```python
from build123d import *

# Parameters (mm, degrees)
SKETCH17_R              = 35
SKETCH18_R              = 60
BOSS_EXTRUDE2_DEPTH     = 10
SKETCH19_R              = 60
BOSS_EXTRUDE3_DEPTH     = 10
CUT_EXTRUDE1_DEPTH      = 153.968934548
CUT_EXTRUDE1_DEPTH_BACK = 10
SKETCH20_R              = 4
SKETCH21_R              = 25
CUT_EXTRUDE3_DEPTH      = 153.968934548
CUT_EXTRUDE3_DEPTH_BACK = 10
SKETCH21_3_R            = 25
SKETCH22_R              = 25
CUT_EXTRUDE10_DEPTH     = 10
CUT_EXTRUDE11_START     = 10
SKETCH22_3_R            = 25
CUT_EXTRUDE11_DEPTH     = 10
SKETCH24_R              = 4
CUT_EXTRUDE18_DEPTH     = 10


with BuildPart() as part:
    # Sweep1: sweep along a path in Sketch16
    with BuildLine(Plane(origin=(0, 0, 0), x_dir=(0, 0, -1), z_dir=(1, 0, 0))) as sweep1_path:
        ThreePointArc((0, 0), (-7.612046749, 38.268343237), (-29.289321881, 70.710678119))
    # Sketch17 → Sweep1 (sweep)
    with BuildSketch(Plane(origin=(0, 0, 0), x_dir=(1, 0, 0), z_dir=(0, 1, 0))):
        with Locations((0, -29.289321881)):
            Circle(SKETCH17_R)
    sweep(path=sweep1_path.line)

    # Sketch18 → Boss-Extrude2 (add)
    with BuildSketch(Plane(origin=(0, 0, 0), x_dir=(-1, 0, 0), z_dir=(0, -1, 0))):
        with Locations(Location((0, -29.289321881, 0), (0, 0, 90))):
            Circle(SKETCH18_R)
    extrude(amount=BOSS_EXTRUDE2_DEPTH)

    # Sketch19 → Boss-Extrude3 (add)
    with BuildSketch(Plane(origin=(0, 50, 50), x_dir=(1, 0, 0), z_dir=(0, 0.7071067811865513, 0.7071067811865438))):
        with Locations(Location((0, 0, 0), (0, 0, 270))):
            Circle(SKETCH19_R)
    extrude(amount=BOSS_EXTRUDE3_DEPTH)

    # Sketch20 → Cut-Extrude1 (cut, two sides: drawn at the far end of the back side and taken through both)
    with BuildSketch(Plane(origin=(0, 0, 0), x_dir=(-1, 0, 0), z_dir=(0, -1, 0)).offset(-CUT_EXTRUDE1_DEPTH_BACK)):
        with Locations(Location((0, 20.710678119, 0), (0, 0, 90))):
            Circle(SKETCH20_R)
        with Locations(Location((25, 14.011948308, 0), (0, 0, 90))):
            Circle(SKETCH20_R)
        with Locations(Location((43.301270189, -4.289321881, 0), (0, 0, 90))):
            Circle(SKETCH20_R)
        with Locations(Location((50, -29.289321881, 0), (0, 0, 90))):
            Circle(SKETCH20_R)
        with Locations(Location((43.301270189, -54.289321881, 0), (0, 0, 90))):
            Circle(SKETCH20_R)
        with Locations(Location((25, -72.590592071, 0), (0, 0, 90))):
            Circle(SKETCH20_R)
        with Locations(Location((0, -79.289321881, 0), (0, 0, 90))):
            Circle(SKETCH20_R)
        with Locations(Location((-25, -72.590592071, 0), (0, 0, 90))):
            Circle(SKETCH20_R)
        with Locations(Location((-43.301270189, -54.289321881, 0), (0, 0, 90))):
            Circle(SKETCH20_R)
        with Locations(Location((-50, -29.289321881, 0), (0, 0, 90))):
            Circle(SKETCH20_R)
        with Locations(Location((-43.301270189, -4.289321881, 0), (0, 0, 90))):
            Circle(SKETCH20_R)
        with Locations(Location((-25, 14.011948308, 0), (0, 0, 90))):
            Circle(SKETCH20_R)
    extrude(amount=CUT_EXTRUDE1_DEPTH + CUT_EXTRUDE1_DEPTH_BACK, mode=Mode.SUBTRACT)

    # Cut-Sweep2: sweep along a path in Sketch16<3>
    with BuildLine(Plane(origin=(0, 0, 0), x_dir=(0, 0, -1), z_dir=(1, 0, 0))) as cut_sweep2_path:
        ThreePointArc((0, 0), (-7.612046749, 38.268343237), (-29.289321881, 70.710678119))
    # Sketch21 → Cut-Sweep2 (sweep, cut)
    with BuildSketch(Plane(origin=(0, 0, 0), x_dir=(-1, 0, 0), z_dir=(0, -1, 0))):
        with Locations((0, -29.289321881)):
            Circle(SKETCH21_R)
    sweep(path=cut_sweep2_path.line, mode=Mode.SUBTRACT)

    # Sketch21<3> → Cut-Extrude3 (cut, two sides: drawn at the far end of the back side and taken through both)
    with BuildSketch(Plane(origin=(0, 0, 0), x_dir=(-1, 0, 0), z_dir=(0, -1, 0)).offset(-CUT_EXTRUDE3_DEPTH_BACK)):
        with Locations(Location((0, -29.289321881, 0), (0, 0, 180.810311696))):
            Circle(SKETCH21_3_R)
    extrude(amount=CUT_EXTRUDE3_DEPTH + CUT_EXTRUDE3_DEPTH_BACK, mode=Mode.SUBTRACT)

    # Sketch22 → Cut-Extrude10 (cut)
    with BuildSketch(Plane(origin=(0, 50, 50), x_dir=(1, 0, 0), z_dir=(0, 0.7071067811865513, 0.7071067811865438))):
        Circle(SKETCH22_R)
    extrude(amount=-CUT_EXTRUDE10_DEPTH, mode=Mode.SUBTRACT)

    # Sketch22<3> → Cut-Extrude11 (cut)
    with BuildSketch(Plane(origin=(0, 50, 50), x_dir=(1, 0, 0), z_dir=(0, 0.7071067811865513, 0.7071067811865438)).offset(CUT_EXTRUDE11_START)):
        with Locations(Location((0, 0, 0), (0, 0, 270))):
            Circle(SKETCH22_3_R)
    extrude(amount=-CUT_EXTRUDE11_DEPTH, mode=Mode.SUBTRACT)

    # Sketch24 → Cut-Extrude18 (cut)
    with BuildSketch(Plane(origin=(0, 50, 50), x_dir=(1, 0, 0), z_dir=(0, 0.7071067811865513, 0.7071067811865438))):
        with Locations(Location((0, 50, 0), (0, 0, 270))):
            Circle(SKETCH24_R)
        with Locations(Location((25, 43.301270189, 0), (0, 0, 270))):
            Circle(SKETCH24_R)
        with Locations(Location((43.301270189, 25, 0), (0, 0, 270))):
            Circle(SKETCH24_R)
        with Locations(Location((50, 0, 0), (0, 0, 270))):
            Circle(SKETCH24_R)
        with Locations(Location((43.301270189, -25, 0), (0, 0, 270))):
            Circle(SKETCH24_R)
        with Locations(Location((25, -43.301270189, 0), (0, 0, 270))):
            Circle(SKETCH24_R)
        with Locations(Location((0, -50, 0), (0, 0, 270))):
            Circle(SKETCH24_R)
        with Locations(Location((-25, -43.301270189, 0), (0, 0, 270))):
            Circle(SKETCH24_R)
        with Locations(Location((-43.301270189, -25, 0), (0, 0, 270))):
            Circle(SKETCH24_R)
        with Locations(Location((-50, 0, 0), (0, 0, 270))):
            Circle(SKETCH24_R)
        with Locations(Location((-43.301270189, 25, 0), (0, 0, 270))):
            Circle(SKETCH24_R)
        with Locations(Location((-25, 43.301270189, 0), (0, 0, 270))):
            Circle(SKETCH24_R)
    extrude(amount=CUT_EXTRUDE18_DEPTH, mode=Mode.SUBTRACT)


solid = part.part
```
Can you work these out from the model? Positions are in its coordinate system, mm. A direction names the side the tool comes from. Round coordinates to 2 decimals unless told otherwise and drop trailing zeros. Loops run counter-clockwise (first coordinate to the right, second up) from the corner with the lowest first, then second, coordinate; pieces in that order, holes last. Notation, with made-up numbers: M 42,18 L 94,18 A11 ccw 94,27 Z; hole C -6.5,81.5 d3. An arc over 180 degrees is marked long. Answer as a JSON object with one key per item and string values. Group by question number.
Q1. Imagine slicing it at B-B, the plane x = -13.5. Please give me the cut outline in (y, z), then the cut area to 3 significant figures.
Q2. We'd pull the mould along X, two halves only. Please class faces 1 (the flat face through (-26, 0, 3)), 2 (the cylindrical face through (-47.206, 71.777, 35.195)): +X half, -X half, draft (parallel to the pull), parting line (faces both ways), or undercut.
Q3. Imagine slicing it at A-A, the plane x = -50. Please give me the cut outline in (y, z), then the cut area to 3 significant figures.
Q4. Imagine slicing it at C-C, the plane z = 56. Count the separate pieces of the cut face and the enclosed holes in it, then the cut area to 3 significant figures.
Q5. On a 3-axis mill with a long thin cutter (end or side, diameter ignored), from which of +Z, -Z, +X, -X, +Y, -Y can I reach the whole of each face in a straight line? I mean faces 3 (the cylindrical face through (-49.824, -4.93, 33.285)), 4 (the cylindrical face through (47.57, 55.73, 51.24)). Say none if no direction works.
Q6. Will these pins go through, and if not, where does the flat tip stop? pin 1 (6.5 mm diameter, centred on x = 50, z = 29.29, fed in from +Y); pin 2 (10.5 mm diameter, centred on x = 0, z = -20.71, fed in from +Y); pin 3 (5 mm diameter, centred on y = 40.5, z = 8, fed in from +X).
Q7. Please list where these lines run through material, in increasing order: L1, parallel to X at y = 43, z = 45; L2, parallel to Z at x = -7, y = 25; L3, parallel to Y at x = 15.5, z = 68.
Findings:
{
 "1": {"outline": "M -10,-29.17 L 0,-29.17 L 0,-3 A103 ccw 72.83,27.17 L 91.34,8.66 L 98.41,15.73 L 71.95,42.19 L 57.81,28.05 L 57.42,28.44 A91.75 cw 10,8.79 L 10,8.25 L -10,8.25 Z; M -10,50.33 L 0,50.33 A49.67 ccw 35.12,64.88 L 42.19,71.95 L 15.73,98.41 L 8.66,91.34 L 27.17,72.83 A38.42 cw 0,61.58 L 0,87.75 L -10,87.75 Z", "area": "2,740 mm2"},
 "2": {"face 1": "draft", "face 2": "undercut"},
 "3": {"outline": "M -10,-3.88 L 0,-3.88 L 0,25.29 L -10,25.29 Z; M -10,33.29 L 0,33.29 L 0,62.46 L -10,62.46 Z; M 26.55,73.45 L 47.17,52.83 L 54.24,59.9 L 33.62,80.52 Z; M 52.83,47.17 L 73.45,26.55 L 80.52,33.62 L 59.9,54.24 Z", "area": "1,170 mm2"},
 "4": {"separate pieces": "3", "enclosed holes": "0", "area": "3,270 mm2"},
 "5": {"face 3": "-Y", "face 4": "none"},
 "6": {"pin 1": "stops at y = 83.33", "pin 2": "stops at y = 0", "pin 3": "stops at x = 21.89"},
 "7": {"L1": "x = -34.99 to -24.98, 24.98 to 34.99", "L2": "z = -1.98 to 8.65, 60.54 to 73.52, 75 to 89.14", "L3": "y = -10 to 0, 22.87 to 40.26"}
}
